```python
from build123d import *

# Parameters (mm, degrees)
F0_W     = 3.9999993443
F0_H     = 48.9999993443
F0_W_2   = 2
F0_H_2   = 47
F1_DEPTH = 25
F2_W     = 43.9999993443
F2_H     = 22.5
F3_DEPTH = 2
F4_DEPTH = 1


# Not quite as in the source:
# - a feature names something its author has since deleted; it is built from what else it names


with BuildPart() as f1:
    # F0 (on Top) → F1 (new body)
    with BuildSketch(Plane.XY):
        with Locations((1.9999996722, 0)):
            Rectangle(F0_W, F0_H)
        with Locations((1.9999996722, 0)):
            Rectangle(F0_W_2, F0_H_2, mode=Mode.SUBTRACT)
    extrude(amount=F1_DEPTH)

    # F2 (on face) → F3 (cut)
    with BuildSketch(Plane.YZ.offset(3.9999993443)):
        with Locations((0, 13.75)):
            Rectangle(F2_W, F2_H)
    extrude(amount=-F3_DEPTH, mode=Mode.SUBTRACT)

    # F0 (on Top) → F4 (join)
    with BuildSketch(Plane.XY):
        with Locations((1.9999996722, 0)):
            Rectangle(F0_W_2, F0_H_2)
    extrude(amount=F4_DEPTH)


solid = f1.part
```
CAD build for the part. Positions are in the model's coordinates, mm. A direction names the side the tool comes from. Coordinates: 2 decimals unless noted, no trailing zeros. Write each loop counter-clockwise with the first axis right and the second up, starting at its lowest first coordinate (ties: lowest second). Pieces come first, ordered by that corner, then holes. Notation, with made-up numbers: (20.25, -20.75) -> (50.25, -20.75) arc R3 ccw to (50.25, -15.75) -> close; hole circle Ø8 at (85.5, 67). An arc over 180 degrees is marked (long way). Return JSON: item names as keys, results as strings. Group by question number.
Q1. Which spindle directions (+Z, -Z, +X, -X, +Y, -Y) get a long thin tool onto all of the face, cutting with end or side? Do faces 5 (the face through (2, 24.5, 12)), 6 (the face through (2, 0, 1)), 7 (the face through (3.5, 22, 13.6)). Say none if no direction does.
Q2. Flat gauge pin, fed straight in: pin 1 (6 mm diameter, centred on y = -17.5, z = 8.5, fed in from +X). Where does the tip first touch, or does it go through?
Q3. Cut at A-A, the plane y = -8. Give the cut face in (x, z), then the cut area to 3 significant figures.
Q4. Pull direction X, two halves, no side cores. Call faces 1 (the face through (4, 0, 2)), 2 (the face through (0, 0, 12)), 3 (the face through (2, -23.5, 13)), 4 (the face through (3.5, -0.3, 2.5)): released by +X, released by -X, zero draft, split by the parting line, or undercut.
Q5. Cut at C-C, the plane x = 2.4. Give the cut face in (y, z), then the cut area to 3 significant figures.
Q6. Cut at B-B, the plane z = 17.75. Give the cut face in (x, y), then the cut area to 3 significant figures.
Q7. Drill centre lines: line 1 (Y direction, x = 3.3, z = 15.75); line 2 (Y direction, x = 2.75, z = 23); line 3 (Z direction, x = 3.35, y = -6.5). Where is each one in solid material? Low to high.
Returned:
{
 "1": {"face 5": "+Z, -Z, +X, -X, +Y", "face 6": "+Z", "face 7": "+Z, +X"},
 "2": {"pin 1": "stops at x = 1"},
 "3": {"outline": "(0, 0) -> (4, 0) -> (4, 2.5) -> (3, 2.5) -> (3, 1) -> (1, 1) -> (1, 25) -> (0, 25) -> close", "area": "29.5 mm2"},
 "4": {"face 1": "released by +X", "face 2": "released by -X", "face 3": "undercut", "face 4": "zero draft"},
 "5": {"outline": "(-24.5, 0) -> (24.5, 0) -> (24.5, 25) -> (23.5, 25) -> (23.5, 1) -> (-23.5, 1) -> (-23.5, 25) -> (-24.5, 25) -> close", "area": "97.0 mm2"},
 "6": {"outline": "(0, -24.5) -> (4, -24.5) -> (4, -22) -> (3, -22) -> (3, -23.5) -> (1, -23.5) -> (1, 23.5) -> (3, 23.5) -> (3, 22) -> (4, 22) -> (4, 24.5) -> (0, 24.5) -> close", "area": "58.0 mm2"},
 "7": {"line 1": "y = -24.5 to -22, 22 to 24.5", "line 2": "y = -24.5 to -23.5, 23.5 to 24.5", "line 3": "z = 0 to 2.5"}
}
